The listing builds one solid part. Answer for the finished solid, in the listing's coordinates (mm). A direction names the side the tool comes from. Round coordinates to 2 decimals unless told otherwise and drop trailing zeros. Write each loop counter-clockwise with the first axis right and the second up, starting at its lowest first coordinate (ties: lowest second). Pieces come first, ordered by that corner, then holes. Notation, with made-up numbers: (71.5, -9.75) - (85.5, -9.75) arc R27 cw to (85.5, 13.25) - close; hole circle Ø9 at (-17, 7). An arc over 180 degrees is marked (long way). Use a Markdown table: item, result. Add a question column.
1) A cutting plane is placed at A-A (y = -39.08). Give the vertices of the cut face in (x, z), then the cut area to 3 significant figures.
2) A cutting plane is placed at D-D (x = -5). Give the vertices of the cut face in (y, z), then the cut area to 3 significant figures.
3) A cutting plane is placed at C-C (y = 9.17). Give the vertices of the cut face in (x, z).
4) Each of these flat-tipped pins is pushed along its axis until it touches: P1, Ø6, axis at x = -7.5, z = -4, coming from the -Y side; P2, Ø3.5, axis at x = -25, z = 5, coming from the +Y side; P3, Ø8, axis at y = -39.5, z = 3, coming from the -X side; P4, Ø2, axis at y = -49, z = 1.5, coming from the -X side. Where does it stop, or does it pass through?
5) Determine the mould class of faces 4 (the flat face through (30, -51.5, 1)), 5 (the cylindrical face through (27.146, 47.951, 5.676)), 6 (the flat face through (-33, 46, 10)) for opening direction Z: +Z half, -Z half, draft (parallel to the pull), parting line (faces both ways), or undercut.
6) A tool of negligible diameter and unlimited length cuts with its end or side. For faces 1 (the flat face through (-34, 36.5, 1)), 2 (the flat face through (26, -48, 6)), 3 (the flat face through (30, -40, 5)), from which of +Z, -Z, +X, -X, +Y, -Y can it reach the whole face along a straight path? Write none if from no direction.
7) Find the intervals of material crossed by probe 1 along Y at (x, z) = (25, 1.5); probe 2 along Y at (x, z) = (-1, -6); probe 3 along X at (y, z) = (-27, -5.75), in increasing order. Write a range as from..to.
8) A cutting plane is placed at B-B (y = 43). Give the vertices of the cut face in (x, z), then the cut area to 4 significant figures.
```python
from build123d import *

# Parameters (mm, degrees)
F0_W     = 7.5
F0_H     = 73
F0_R     = 2.25
F1_DEPTH = 7.5
F2_DEPTH = 10
F3_R     = 2.25
F4_DEPTH = 75
F5_SIZE  = 7.5
F6_R     = 5


with BuildPart() as f1:
    # F0 (on Top) → F1 (new body)
    with BuildSketch(Plane.XY):
        with Locations((33.75, 0)):
            Rectangle(F0_W, F0_H)
        Polygon((37.5, -51.5), (37.5, -36.5), (30, -36.5), (30, -44), (22.5, -44), (22.5, -51.5), align=None)
        Polygon((30, 44.5), (20, 44.5), (17.5, 44.5), (17.5, 31.5), (17.5, -44.014243), (22.5, -51.5), (22.5, -44), (30, -44), (30, -36.5), (30, 36.5), align=None)
        with Locations((24.92, -39.08)):
            Circle(F0_R, mode=Mode.SUBTRACT)
        with Locations((24.92, 9.17)):
            Circle(F0_R, mode=Mode.SUBTRACT)
        Polygon((37.5, 51.5), (20, 51.5), (20, 44.5), (30, 44.5), (30, 36.5), (37.5, 36.5), align=None)
        Polygon((20, 51.5), (-20, 51.5), (-20, 44.5), (17.5, 44.5), (20, 44.5), align=None)
        Polygon((-20, 51.5), (-37.5, 51.5), (-37.5, 36.5), (-30, 36.5), (-30, 44.5), (-20, 44.5), align=None)
        Polygon((17.5, 44.5), (-20, 44.5), (-30, 44.5), (-30, 36.5), (-22.5, 31.5), (17.5, 31.5), align=None)
    extrude(amount=-F1_DEPTH)

    # F0 (on Top) → F2 (join)
    with BuildSketch(Plane.XY):
        Polygon((37.5, 51.5), (20, 51.5), (20, 44.5), (30, 44.5), (30, 36.5), (37.5, 36.5), align=None)
        Polygon((37.5, -51.5), (37.5, -36.5), (30, -36.5), (30, -44), (22.5, -44), (22.5, -51.5), align=None)
        Polygon((-20, 51.5), (-37.5, 51.5), (-37.5, 36.5), (-30, 36.5), (-30, 44.5), (-20, 44.5), align=None)
    extrude(amount=F2_DEPTH)

    # F3 (on Front) → F4 (cut)
    with BuildSketch(Plane.XZ):
        with Locations((25, 5)):
            Circle(F3_R)
        with Locations((-25, 5)):
            Circle(F3_R)
    extrude(amount=-F4_DEPTH, mode=Mode.SUBTRACT)

    # F5
    f5_edges = [f1.edges().sort_by_distance(p)[0] for p in [
        (22.5, -47.75, 10),
    ]]
    chamfer(f5_edges, length=F5_SIZE)

    # F6
    f6_edges = [f1.edges().sort_by_distance(p)[0] for p in [
        (-20, 48, 10),
        (20, 48, 10),
    ]]
    fillet(f6_edges, radius=F6_R)


solid = f1.part
```
Entries:
| question | item | result |
|---|---|---|
| 1 | outline | (17.5, -7.5) - (22.67, -7.5) - (22.67, 0) - (17.5, 0) - close; (27.17, -7.5) - (37.5, -7.5) - (37.5, 10) - (30, 10) - (30, 0) - (27.17, 0) - close |
| 1 | area | 191 mm² |
| 2 | outline | (31.5, -7.5) - (51.5, -7.5) - (51.5, 0) - (31.5, 0) - close |
| 2 | area | 150 mm² |
| 3 | outline | (17.5, -7.5) - (22.67, -7.5) - (22.67, 0) - (17.5, 0) - close; (27.17, -7.5) - (37.5, -7.5) - (37.5, 0) - (27.17, 0) - close |
| 4 | P1 | stops at y = 31.5 |
| 4 | P2 | passes through |
| 4 | P3 | stops at x = 17.5 |
| 4 | P4 | stops at x = 22.5 |
| 5 | face 4 | draft |
| 5 | face 5 | undercut |
| 5 | face 6 | +Z half |
| 6 | face 1 | +Z, -Z, -X, -Y |
| 6 | face 2 | +Z, -X, -Y |
| 6 | face 3 | +Z, -X |
| 7 | probe 1 | y = -51.5..-44, 44.5..51.5 |
| 7 | probe 2 | y = 31.5..51.5 |
| 7 | probe 3 | x = 17.5..37.5 |
| 8 | outline | (-37.5, -7.5) - (37.5, -7.5) - (37.5, 10) - (30, 10) - (30, 0) - (-30, 0) - (-30, 10) - (-37.5, 10) - close |
| 8 | area | 712.5 mm² |
